The model under review builds one solid part; all positions refer to its coordinate system, in mm. Round coordinates to 2 decimals unless told otherwise and drop trailing zeros. Loops run counter-clockwise (first coordinate to the right, second up) from the corner with the lowest first, then second, coordinate; pieces in that order, holes last. Notation, with made-up numbers: M -39,17 L -34,17 A10 cw -34,23 Z; hole C 41.25,7.5 d2. An arc over 180 degrees is marked long. Return JSON: item names as keys, results as strings. Group by question number.
Q1. Consider section D-D (y = 2.5). State the section outline as (x, z) points, and give its area (3 significant figures).
Q2. Consider section C-C (z = 0.2). Count the separate pieces of the cut face and the enclosed holes in it, and give its area (3 significant figures).
Q3. Consider section A-A (y = -11.5). State the section outline as (x, z) points.
Q4. Draft analysis for pull direction Y (two halves, no side actions). For faces 1 (the face through (0, 0, 1.2)), 2 (the face through (0, 14, 1)), 3 (the face through (26.3, 11.43, 0.61)), state which applies: pulls with the +Y half, pulls with the -Y half, needs draft (parallel to the pull), parting line crosses it, or undercut.
Q5. Consider section B-B (x = 24.3). State the section outline as (y, z) points.
Q6. To check wall thickness, follow line 1 along X through (y, z) = (2, 1.05); line 2 along X through (y, z) = (-12.5, 0.2); line 3 along Y through (x, z) = (24.8, 0.45). State the ranges of each line that lie inside material, in increasing order.
from build123d import *

# Parameters (mm, degrees)
ESBO_O1_W                = 54.6
ESBO_O1_H                = 28
RESSALTO_EXTRUS_O1_DEPTH = 1.2
ESBO_O2_R                = 1.5
CORTE_EXTRUS_O1_DEPTH    = 31.703908546
ESBO_O3_R                = 0.75
CORTE_EXTRUS_O2_DEPTH    = 31.703908546


with BuildPart() as part:
    # Esboço1 → Ressalto-extrusão1 (new body)
    with BuildSketch(Plane.XY):
        Rectangle(ESBO_O1_W, ESBO_O1_H)
    extrude(amount=RESSALTO_EXTRUS_O1_DEPTH)

    # Esboço2 → Corte-extrusão1 (cut, through all)
    with BuildSketch(Plane.XY.offset(1.2)):
        with Locations((-24.8, 11.5)):
            Circle(ESBO_O2_R)
        with Locations(Location((24.8, 11.5, 0), (0, 0, 180))):
            Circle(ESBO_O2_R)
        with Locations(Location((-24.8, -11.5, 0), (0, 0, 180))):
            Circle(ESBO_O2_R)
        with Locations((24.8, -11.5)):
            Circle(ESBO_O2_R)
    extrude(amount=-CORTE_EXTRUS_O1_DEPTH, mode=Mode.SUBTRACT)

    # Esboço3 → Corte-extrusão2 (cut, through all)
    with BuildSketch(Plane.XY.offset(1.2)):
        with Locations((24.3, 2.5)):
            Circle(ESBO_O3_R)
        with Locations(Location((24.3, -2.5, 0), (0, 0, 180))):
            Circle(ESBO_O3_R)
        with Locations((-24.3, -2.5)):
            Circle(ESBO_O3_R)
        with Locations(Location((-24.3, 2.5, 0), (0, 0, 180))):
            Circle(ESBO_O3_R)
    extrude(amount=-CORTE_EXTRUS_O2_DEPTH, mode=Mode.SUBTRACT)


solid = part.part
Values:
{
 "1": {"outline": "M -27.3,0 L -25.05,0 L -25.05,1.2 L -27.3,1.2 Z; M -23.55,0 L 23.55,0 L 23.55,1.2 L -23.55,1.2 Z; M 25.05,0 L 27.3,0 L 27.3,1.2 L 25.05,1.2 Z", "area": "61.9 mm2"},
 "2": {"separate pieces": "1", "enclosed holes": "8", "area": "1,490 mm2"},
 "3": {"outline": "M -27.3,0 L -26.3,0 L -26.3,1.2 L -27.3,1.2 Z; M -23.3,0 L 23.3,0 L 23.3,1.2 L -23.3,1.2 Z; M 26.3,0 L 27.3,0 L 27.3,1.2 L 26.3,1.2 Z"},
 "4": {"face 1": "needs draft", "face 2": "pulls with the +Y half", "face 3": "undercut"},
 "5": {"outline": "M -14,0 L -12.91,0 L -12.91,1.2 L -14,1.2 Z; M -10.09,0 L -3.25,0 L -3.25,1.2 L -10.09,1.2 Z; M -1.75,0 L 1.75,0 L 1.75,1.2 L -1.75,1.2 Z; M 3.25,0 L 10.09,0 L 10.09,1.2 L 3.25,1.2 Z; M 12.91,0 L 14,0 L 14,1.2 L 12.91,1.2 Z"},
 "6": {"line 1": "x = -27.3 to -24.86, -23.74 to 23.74, 24.86 to 27.3", "line 2": "x = -27.3 to -25.92, -23.68 to 23.68, 25.92 to 27.3", "line 3": "y = -14 to -13, -10 to -3.06, -1.94 to 1.94, 3.06 to 10, 13 to 14"}
}
